CAD build for the part. Positions are in the model's coordinates, mm. Face numbers are marked on the shaded views. Round coordinates to 2 decimals unless told otherwise and drop trailing zeros. Order: outer loops, then holes, each group sorted by start corner. A loop starts at its lowest first (then second) coordinate and runs counter-clockwise, first axis right, second up. Notation, with made-up numbers: (45.5, 4.25) -> (81.5, 4.25) arc R19 ccw to (81.5, 21.25) -> close; hole circle Ø8 at (50, 41.25). An arc over 180 degrees is marked (long way). Return JSON: item names as keys, results as strings. Group by question number.
Q1. Cut at A-A (y = 0). Write the cut outline in (x, z), then the cut area to 3 significant figures.
Q2. Flat gauge pin, fed straight in: pin 1 (1 mm diameter, centred on y = 4.5, z = 0.5, fed in from +X). Where does the tip first touch, or does it go through?
Q3. Probe line 1 along X through (y, z) = (-10, 3.3); line 2 along Y through (x, z) = (0.5, 3.65). List the from-to ranges inside material, lowest first.
Q4. Cut at D-D (x = -8). Write the cut outline in (y, z), then the cut area to 3 significant figures.
Q5. Cut at C-C (z = 1.55). Count the separate pieces of the cut face and the enclosed holes in it, then the cut area to 3 significant figures.
Q6. Cut at B-B (x = -2). Write the cut outline in (y, z).
Q7. Mould opens along X. For the marked faces 1, 2 and 3 say: +X half, -X half, draft (parallel to the pull), parting line (faces both ways), or undercut.
Solid Edge part; units mm, degrees
sketch "Sketch1" plane through (0, 0, 0) normal (0, 0, 1) x (1, 0, 0)
  circle A0 centre (0, 0) radius 17
  circle A1 centre (0, 0) radius 4
  circle A2 centre (8, 0) radius 1.15
  circle A3 centre (0, 8) radius 1.15
  circle A4 centre (-8, 0) radius 1.15
  circle A5 centre (0, -8) radius 1.15
  circle A6 centre (9.1924, 9.1924) radius 1.7
  circle A7 centre (-9.1924, 9.1924) radius 1.7
  circle A8 centre (-9.1924, -9.1924) radius 1.7
  circle A9 centre (9.1924, -9.1924) radius 1.7
extrude "Protrusion1" add sketch "Sketch1" along normal blind 4
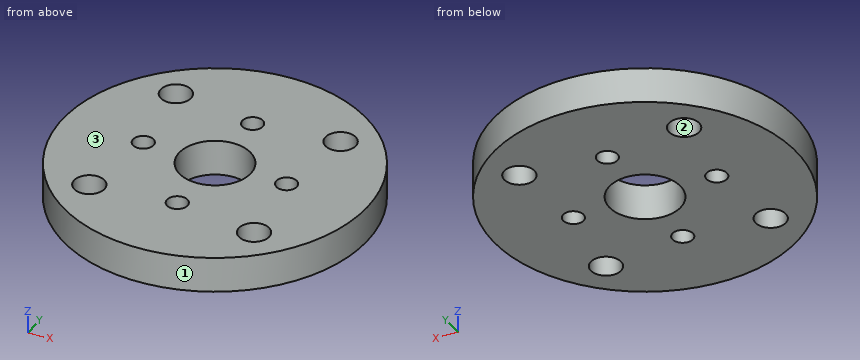
Solution:
{
 "1": {"outline": "(-17, 0) -> (-9.15, 0) -> (-9.15, 4) -> (-17, 4) -> close; (-6.85, 0) -> (-4, 0) -> (-4, 4) -> (-6.85, 4) -> close; (4, 0) -> (6.85, 0) -> (6.85, 4) -> (4, 4) -> close; (9.15, 0) -> (17, 0) -> (17, 4) -> (9.15, 4) -> close", "area": "85.6 mm²"},
 "2": {"pin 1": "stops at x = 16.52"},
 "3": {"line 1": "x = -13.75 to -10.69, -7.7 to 7.7, 10.69 to 13.75", "line 2": "y = -16.99 to -9.04, -6.96 to -3.97, 3.97 to 6.96, 9.04 to 16.99"},
 "4": {"outline": "(-15, 0) -> (-10.4, 0) -> (-10.4, 4) -> (-15, 4) -> close; (-7.98, 0) -> (-1.15, 0) -> (-1.15, 4) -> (-7.98, 4) -> close; (1.15, 0) -> (7.98, 0) -> (7.98, 4) -> (1.15, 4) -> close; (10.4, 0) -> (15, 0) -> (15, 4) -> (10.4, 4) -> close", "area": "91.4 mm²"},
 "5": {"separate pieces": "1", "enclosed holes": "9", "area": "805 mm²"},
 "6": {"outline": "(-16.88, 0) -> (-3.46, 0) -> (-3.46, 4) -> (-16.88, 4) -> close; (3.46, 0) -> (16.88, 0) -> (16.88, 4) -> (3.46, 4) -> close"},
 "7": {"face 1": "parting line", "face 2": "undercut", "face 3": "draft"}
}
